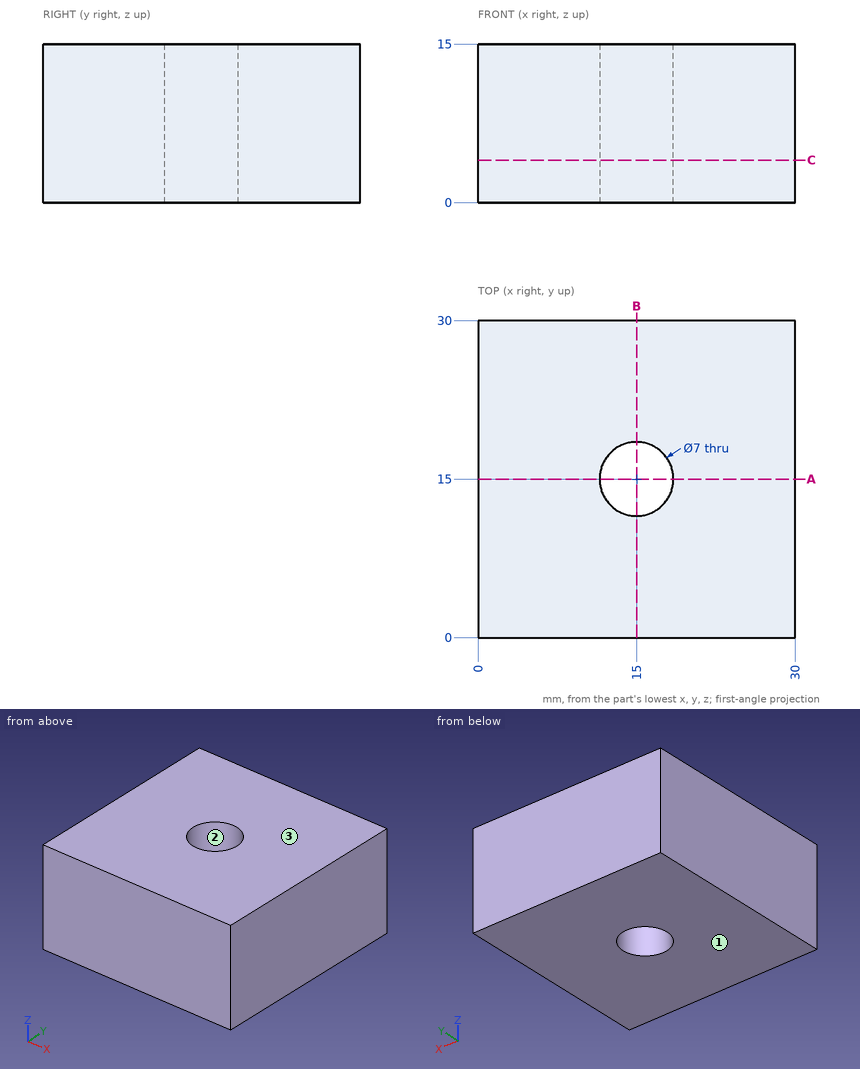
Could you check a few things on this drawing? It's one solid part, dimensions in mm from its lowest x, y, z. Coordinates: 2 decimals unless noted, no trailing zeros. Order: outer loops, then holes, each group sorted by start corner. A loop starts at its lowest first (then second) coordinate and runs counter-clockwise, first axis right, second up. Notation, with made-up numbers: (50, 6.25) - (80, 6.25) arc R13 cw to (80, 18.25) - close; hole circle Ø8 at (2.5, -11). An arc over 180 degrees is marked (long way). Answer as a JSON object with one key per item and string values. Group by question number.
Q1. Imagine slicing it at A-A (y = 15). Please give me the cut outline in (x, z), and give its area (3 significant figures).
Q2. I need wall thicknesses on line 1 (X direction, y = 15, z = 4.75); line 2 (X direction, y = 14.25, z = 11.75). Which ranges of each line are inside material? Lowest first, please. Write a range as from..to.
Q3. We'd pull the mould along Z, two halves only. Please class the marked faces 1, 2 and 3: +Z half, -Z half, draft (parallel to the pull), parting line (faces both ways), or undercut.
Q4. Imagine slicing it at C-C (z = 4). Please give me the cut outline in (x, y), and give its area (3 significant figures).
Determined:
{
 "1": {"outline": "(0, 0) - (11.5, 0) - (11.5, 15) - (0, 15) - close; (18.5, 0) - (30, 0) - (30, 15) - (18.5, 15) - close", "area": "345 mm2"},
 "2": {"line 1": "x = 0..11.5, 18.5..30", "line 2": "x = 0..11.58, 18.42..30"},
 "3": {"face 1": "-Z half", "face 2": "draft", "face 3": "+Z half"},
 "4": {"outline": "(0, 0) - (30, 0) - (30, 30) - (0, 30) - close; hole circle Ø7 at (15, 15)", "area": "862 mm2"}
}
